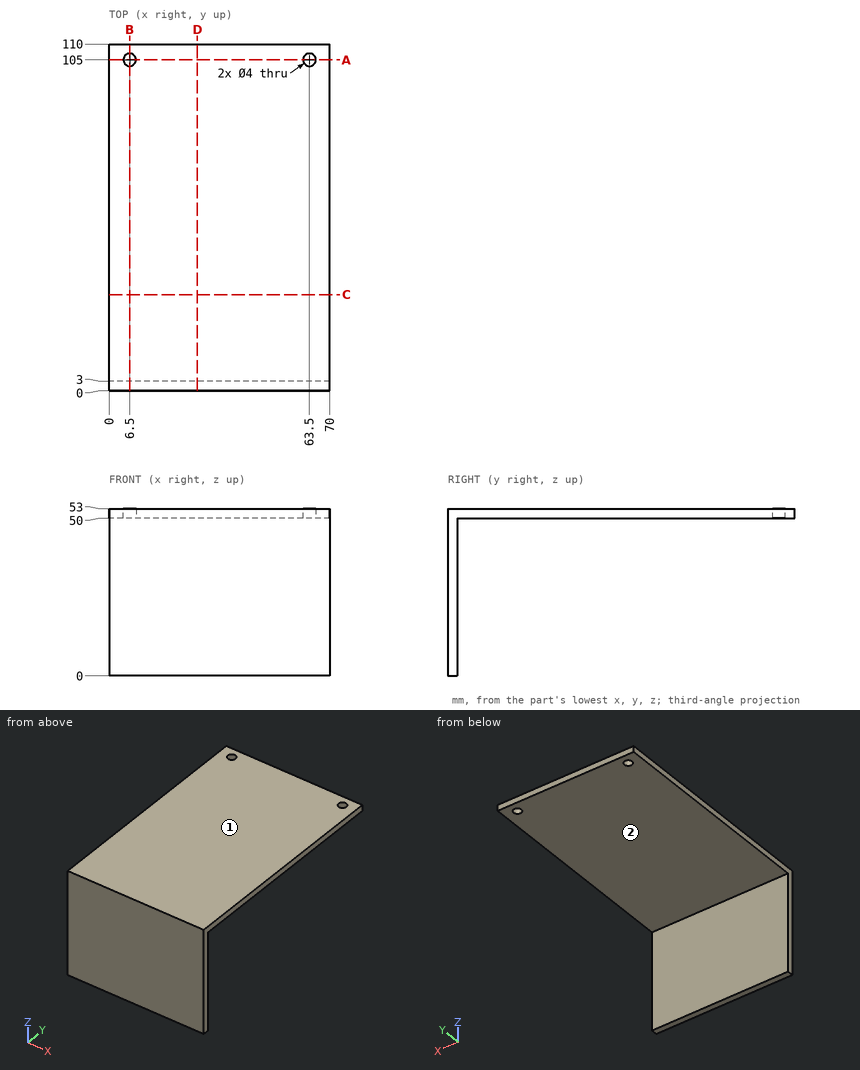
Geometry: see drawing. Coordinates: mm, zero at the bounding-box minimum. A direction names the side the tool comes from. Coordinates: 2 decimals unless noted, no trailing zeros. Write each loop counter-clockwise with the first axis right and the second up, starting at its lowest first coordinate (ties: lowest second). Pieces come first, ordered by that corner, then holes.
1) Set-up query: the marked faces 1 and 2. Return all of +Z, -Z, +X, -X, +Y, -Y with unobstructed straight access to the full face (end or side cutting, diameter ignored); none if empty.
2) Section C-C on y = 30.5. Output: boundary loops of the cut face in (x, z), and give its area (3 significant figures).
3) Pin query (flat end, axial travel): pin 1 Ø8 at (x, y) = (36.5, 78.5) entering from -Z; pin 2 Ø5 at (x, z) = (26.5, 15) entering from +Y; pin 3 Ø10 at (x, z) = (44, 43.5) entering from -Y. Return the tip coordinate at first contact, or that it passes through.
4) Section A-A on y = 105. Output: boundary loops of the cut face in (x, z).
5) Material intervals for line 1 along X through (y, z) = (105, 51.95); line 2 along Y through (x, z) = (63.5, 50.95); line 3 along Z through (x, y) = (46.5, 22), sorted ascending.
6) Section B-B on x = 6.5. Output: boundary loops of the cut face in (y, z), and give its area (3 significant figures).
7) Section D-D on x = 28. Output: boundary loops of the cut face in (y, z).
Check result:
1. face 1: +Z, +X, -X, +Y, -Y
1. face 2: -Z, +X, -X, +Y
2. outline: (0, 50) - (70, 50) - (70, 53) - (0, 53) - close
2. area: 210 mm2
3. pin 1: stops at z = 50
3. pin 2: stops at y = 3
3. pin 3: stops at y = 0
4. outline: (0, 50) - (4.5, 50) - (4.5, 53) - (0, 53) - close; (8.5, 50) - (61.5, 50) - (61.5, 53) - (8.5, 53) - close; (65.5, 50) - (70, 50) - (70, 53) - (65.5, 53) - close
5. line 1: x = 0 to 4.5, 8.5 to 61.5, 65.5 to 70
5. line 2: y = 0 to 103, 107 to 110
5. line 3: z = 50 to 53
6. outline: (0, 0) - (3, 0) - (3, 50) - (103, 50) - (103, 53) - (0, 53) - close; (107, 50) - (110, 50) - (110, 53) - (107, 53) - close
6. area: 468 mm2
7. outline: (0, 0) - (3, 0) - (3, 50) - (110, 50) - (110, 53) - (0, 53) - close
